Source: CAD feature listing. Evaluate the final solid. Frame: model axes, mm. Coordinates: 2 decimals unless noted, no trailing zeros. Write each loop counter-clockwise with the first axis right and the second up, starting at its lowest first coordinate (ties: lowest second). Pieces come first, ordered by that corner, then holes. Notation, with made-up numbers: (78, 60.25) - (116, 60.25) arc R14 cw to (116, 77.25) - close; hole circle Ø10 at (76, -36). An arc over 180 degrees is marked (long way). One line per item, written item: value.
from build123d import *

# Parameters (mm, degrees)
F0_R     = 11
F1_DEPTH = 6
F2_SIZE  = 1


with BuildPart() as f1:
    # F0 (on Top) → F1 (new body)
    with BuildSketch(Plane.XY):
        with BuildLine():
            ThreePointArc((-11.139458, 19.548976), (-11.667262, 11.667262), (-19.548976, 11.139458))
            ThreePointArc((-19.548976, 11.139458), (-20.787289, 8.610377), (-21.7, 5.946427))
            ThreePointArc((-21.7, 5.946427), (-16.5, 0), (-21.7, -5.946427))
            ThreePointArc((-21.7, -5.946427), (-20.787289, -8.610377), (-19.548976, -11.139458))
            ThreePointArc((-19.548976, -11.139458), (-11.667262, -11.667262), (-11.139458, -19.548976))
            ThreePointArc((-11.139458, -19.548976), (-8.610377, -20.787289), (-5.946427, -21.7))
            ThreePointArc((-5.946427, -21.7), (0, -16.5), (5.946427, -21.7))
            ThreePointArc((5.946427, -21.7), (8.610377, -20.787289), (11.139458, -19.548976))
            ThreePointArc((11.139458, -19.548976), (11.667262, -11.667262), (19.548976, -11.139458))
            ThreePointArc((19.548976, -11.139458), (20.787289, -8.610377), (21.7, -5.946427))
            ThreePointArc((21.7, -5.946427), (16.5, 0), (21.7, 5.946427))
            ThreePointArc((21.7, 5.946427), (20.787289, 8.610377), (19.548976, 11.139458))
            ThreePointArc((19.548976, 11.139458), (11.667262, 11.667262), (11.139458, 19.548976))
            ThreePointArc((11.139458, 19.548976), (8.610377, 20.787289), (5.946427, 21.7))
            ThreePointArc((5.946427, 21.7), (0, 16.5), (-5.946427, 21.7))
            ThreePointArc((-5.946427, 21.7), (-8.610377, 20.787289), (-11.139458, 19.548976))
        make_face()
        Circle(F0_R, mode=Mode.SUBTRACT)
    extrude(amount=F1_DEPTH)

    # F2
    f2_edges = [f1.edges().sort_by_distance(p)[0] for p in [
        (-16.5, 0, 0),
        (-20.787289, 8.610377, 0),
        (-11.667262, 11.667262, 0),
        (-8.610377, 20.787289, 0),
        (0, 16.5, 0),
        (8.610377, 20.787289, 0),
        (11.667262, 11.667262, 0),
        (20.787289, 8.610377, 0),
        (16.5, 0, 0),
        (11.667262, -11.667262, 0),
        (20.787289, -8.610377, 0),
        (8.610377, -20.787289, 0),
        (0, -16.5, 0),
        (-8.610377, -20.787289, 0),
        (-11.667262, -11.667262, 0),
        (-20.787289, -8.610377, 0),
        (0, 16.5, 6),
        (-11.667262, 11.667262, 6),
        (-8.610377, 20.787289, 6),
        (8.610377, 20.787289, 6),
        (11.667262, 11.667262, 6),
        (20.787289, 8.610377, 6),
        (16.5, 0, 6),
        (20.787289, -8.610377, 6),
        (11.667262, -11.667262, 6),
        (0, -16.5, 6),
        (8.610377, -20.787289, 6),
        (-8.610377, -20.787289, 6),
        (-11.667262, -11.667262, 6),
        (-20.787289, -8.610377, 6),
        (-16.5, 0, 6),
        (-20.787289, 8.610377, 6),
    ]]
    chamfer(f2_edges, length=F2_SIZE)


solid = f1.part
1) Material intervals for line 1 (X direction, y = -10, z = 0.5); line 2 (X direction, y = 3.5, z = 5); line 3 (X direction, y = -1.5, z = 0.75), sorted ascending.
Values found:
line 1: -19.6 to -18.62, -13.2 to -4.58, 4.58 to 13.2, 18.62 to 19.6
line 2: -17.63 to -10.43, 10.43 to 17.63
line 3: -16.43 to -10.9, 10.9 to 16.43
2) Section query D-D on z = 5.5. Output: boundary loops of the cut face in (x, y), then the cut area to 3 significant figures.
Values found:
outline: (-21.07, -6.34) arc R22 ccw to (-19.38, -10.41) arc R6.5 cw to (-10.41, -19.38) arc R22 ccw to (-6.34, -21.07) arc R6.5 cw to (6.34, -21.07) arc R22 ccw to (10.41, -19.38) arc R6.5 cw to (19.38, -10.41) arc R22 ccw to (21.07, -6.34) arc R6.5 cw to (21.07, 6.34) arc R22 ccw to (19.38, 10.41) arc R6.5 cw to (10.41, 19.38) arc R22 ccw to (6.34, 21.07) arc R6.5 cw to (-6.34, 21.07) arc R22 ccw to (-10.41, 19.38) arc R6.5 cw to (-19.38, 10.41) arc R22 ccw to (-21.07, 6.34) arc R6.5 cw to start; hole circle Ø22 at (0, 0)
area: 694 mm2
3) Contact query for flat-ended pins moving along their axis: P1, Ø1, axis at y = -12.5, z = 4.5, coming from the +X side; P2, Ø2, axis at x = 8.5, z = 4, coming from the -Y side. Output: stop coordinate, or through.
Values found:
P1: x = 11.36
P2: y = -21.21
4) Section query C-C on z = 2. Output: boundary loops of the cut face in (x, y).
Values found:
outline: (-21.7, -5.95) arc R22.5 ccw to (-19.55, -11.14) arc R6 cw to (-11.14, -19.55) arc R22.5 ccw to (-5.95, -21.7) arc R6 cw to (5.95, -21.7) arc R22.5 ccw to (11.14, -19.55) arc R6 cw to (19.55, -11.14) arc R22.5 ccw to (21.7, -5.95) arc R6 cw to (21.7, 5.95) arc R22.5 ccw to (19.55, 11.14) arc R6 cw to (11.14, 19.55) arc R22.5 ccw to (5.95, 21.7) arc R6 cw to (-5.95, 21.7) arc R22.5 ccw to (-11.14, 19.55) arc R6 cw to (-19.55, 11.14) arc R22.5 ccw to (-21.7, 5.95) arc R6 cw to start; hole circle Ø22 at (0, 0)
5) Section query A-A on y = 0. Output: boundary loops of the cut face in (x, z).
Values found:
outline: (-16.5, 1) - (-15.5, 0) - (-11, 0) - (-11, 6) - (-15.5, 6) - (-16.5, 5) - close; (11, 0) - (15.5, 0) - (16.5, 1) - (16.5, 5) - (15.5, 6) - (11, 6) - close
6) Draft query along X for faces 1 (the conical face through (11.458, -11.633, 5.174)), 2 (the cylindrical face through (11.583, -11.753, 2.972)), 3 (the cylindrical face through (-8.574, 20.802, 2.972)), 4 (the cylindrical face through (20.802, 8.574, 2.972)). Return one class per face: released by +X, released by -X, zero draft, split by the parting line, or undercut.
Values found:
face 1: undercut
face 2: undercut
face 3: released by -X
face 4: released by +X
